The model under review builds one solid part; all positions refer to its coordinate system, in mm. A direction names the side the tool comes from. Round coordinates to 2 decimals unless told otherwise and drop trailing zeros. Order: outer loops, then holes, each group sorted by start corner. A loop starts at its lowest first (then second) coordinate and runs counter-clockwise, first axis right, second up. Notation, with made-up numbers: (-10, 71.5) - (39, 71.5) arc R10 cw to (39, 89.5) - close; hole circle Ø5 at (-29.5, -39). An arc over 180 degrees is marked (long way). One line per question, with ' | ' between items. Start each with the question number.
Item 1: For L1, parallel to Y at x = 88, z = 0.75; L2, parallel to X at y = 5, z = 1.3; L3, parallel to X at y = 3, z = 2.65, list the stretches that pass through material, from the lowest coordinate up. Write a range as [from, to].
Item 2: Tool access review of faces 1 (the face through (48, 40, 2)), 2 (the face through (37, 24, 0)), 3 (the face through (55, 20, 4)), 4 (the face through (78, 10, 2)): name each direction out of +Z, -Z, +X, -X, +Y, -Y from which nothing blocks a thin tool from reaching the whole face with its end or side.
Item 3: Add section B-B on z = 4.05. State the section outline as (x, y) points (3 decimals), and give its area (3 significant figures).
Item 4: Draft analysis for pull direction Y (two halves, no side actions). For faces 5 (the face through (13, 60, 2)), 6 (the face through (37, 24, 5)), 7 (the face through (89.3, 18.7, 2)), state which applies: +Y half, -Y half, draft (parallel to the pull), parting line (faces both ways), or undercut.
Item 5: Add section D-D on x = 54. State the section outline as (y, z) points, and give its area (3 significant figures).
Item 6: Add section C-C on y = 20. State the section outline as (x, z) points (3 decimals).
Item 7: Insertion check: pin 1 Ø1 at (x, z) = (87.5, 2.5) entering from -Y; pin 2 Ø2 at (y, z) = (20.5, 1.5) entering from -X; pin 3 Ø1.5 at (y, z) = (36, 1.5) entering from +X; pin 4 Ø1.9 at (x, y) = (88, 20) entering from -Z. Each pin has a flat end and moves straight along its axis. Give the tip position at first contact, or say it passes through.
Item 8: Add section A-A on x = 88. State the section outline as (y, z) points.
Autodesk Inventor part; units mm, degrees
ref_plane "YZ Plane" through (0, 0, 0) normal (1, 0, 0) x (0, 1, 0)
ref_plane "XZ Plane" through (0, 0, 0) normal (0, 1, 0) x (-1, 0, 0)
ref_plane "XY Plane" through (0, 0, 0) normal (0, 0, 1) x (1, 0, 0)
sketch "スケッチ1" plane through (0, 0, 0) normal (0, 0, 1) x (1, 0, 0)
  line L0 (0, 0) -> (98, 0)
  line L1 (98, 0) -> (98, 60)
  line L2 (98, 60) -> (0, 60)
  line L3 (0, 60) -> (0, 0)
  line L4 (98, 0) -> (29, 0)
  line L5 (29, 0) -> (29, 40)
  line L6 (29, 40) -> (98, 40)
  line L7 (98, 40) -> (98, 0)
  line L8 (29, 30) -> (98, 30)
  line L9 (98, 30) -> (98, 10)
  line L10 (98, 10) -> (29, 10)
  line L11 (29, 10) -> (29, 30)
  line L12 (98, 20) -> (0, 20)
  line L13 (29, 20) -> (5.906, 60)
  circle A0 centre (29, 20) radius 8.025
  circle A1 centre (14, 45.9808) radius 4.025
  line L14 (58, 40) -> (58, 0)
  line L15 (16.8756, 13) -> (-6.2184, 53)
  line L16 (41.1244, 27) -> (18.0303, 67)
  circle A2 centre (14, 45.9808) radius 14
  line L17 (16.8756, 13) -> (25.3526, -1.6825)
  point P0 (58, 30)
  point P1 (33.6188, 40)
  point P2 (22.0718, 60)
  point P3 (0, 45.9808)
  point P4 (1.8756, 38.9808)
  point P5 (24.3812, 0)
  point P6 (58, 0)
  point P7 (58, 10)
  dimension "d0" = 98
  dimension "d1" = 60
  dimension "d2" = 40
  dimension "d3" = 20
  dimension "d4" = 10
  dimension "d5" = 69
  dimension "d6" = 30
  dimension "d7" = 16.05
  dimension "d8" = 30
  dimension "d9" = 8.05
  dimension "d10" = 40
  dimension "d11" = 28
extrude "押し出し1" add sketch "スケッチ1" along normal blind 5 contours L5 L10 L14 L0 | L0 L17 L15 L12 A0 L5 | L5 A0 L12 L14 L10 | L14 L12 L1 L10 | L14 L8 L1 L12 | L12 A0 L5 L8 L14 | L15 A2 L13 A0 L12 | L8 L16 L6 L14 | A2 L13 A1 | A0 L13 A2 L16 L6 L5 | L8 L5 L6 L16 | L3 L2 L13 A2 | L13 A1 A2 | L13 L2 L16 A2
sketch "スケッチ2" plane through (0, 0, 5) normal (0, 0, 1) x (1, 0, 0)
  line L0 (98, 10) -> (98, 30)
  line L1 (98, 20) -> (47.1161, 20)
  point P0 (0, 0)
  point P1 (88, 20)
  point P2 (58, 20)
  dimension "d14" = 10
  dimension "d15" = 30
hole "穴1" at (88, 20, 5) at (58, 20, 5) direction (0, 0, -1) diameter 3.2 depth 10
fillet "フィレット1" radius 2 6 edges at (58, 40, 2.5) (58, 30, 2.5) (98, 30, 2.5) (98, 10, 2.5) (58, 0, 2.5) (58, 10, 2.5)
fillet "フィレット2" radius 10 4 edges at (24.3812, 0, 2.5) (0, 60, 2.5) (22.0718, 60, 2.5) (33.6188, 40, 2.5)
sketch "スケッチ4" plane through (0, 0, 5) normal (0, 0, 1) x (1, 0, 0)
  circle A0 centre (58, 20) radius 1.6
  circle A1 centre (58, 20) radius 3
  circle A2 centre (88, 20) radius 1.6
  circle A3 centre (88, 20) radius 3
  point P0 (0, 0)
  dimension "d34" = 6
  dimension "d35" = 6
extrude "押し出し2" cut sketch "スケッチ4" against normal blind 3 contours A0 | A1 | A2 | A3
equation "\"d35\" = d34"
properties part number "RP_Calf-Link-cover-Outside-Right"
Determined:
1) L1: [10, 18.4], [21.6, 30] | L2: [21.49, 58] | L3: [23.01, 58]
2) face 1: +Z, -Z, +X, +Y | face 2: -Z, +X, -X, +Y, -Y | face 3: +Z | face 4: +Z, -Z, +X, -Y
3) outline: (0, 45.981) arc R14 ccw to (1.876, 38.981) - (16.876, 13) - (21.494, 5) arc R10 ccw to (30.155, 0) - (56, 0) arc R2 ccw to (58, 2) - (58, 8) arc R2 cw to (60, 10) - (96, 10) arc R2 ccw to (98, 12) - (98, 28) arc R2 ccw to (96, 30) - (60, 30) arc R2 cw to (58, 32) - (58, 38) arc R2 ccw to (56, 40) - (39.392, 40) arc R10 cw to (30.732, 45) - (24.959, 55) arc R10 ccw to (16.298, 60) - (10, 60) arc R10 ccw to (0, 50) - close; hole circle Ø8.05 at (14, 45.981); hole circle Ø16.05 at (29, 20); hole circle Ø6 at (58, 20); hole circle Ø6 at (88, 20) | area: 2,820 mm2
4) face 5: +Y half | face 6: draft | face 7: undercut
5) outline: (0, 0) - (40, 0) - (40, 5) - (0, 5) - close | area: 200 mm2
6) outline: (12.834, 0) - (20.975, 0) - (20.975, 5) - (12.834, 5) - close; (37.025, 0) - (56.4, 0) - (56.4, 2) - (55, 2) - (55, 5) - (37.025, 5) - close; (59.6, 0) - (86.4, 0) - (86.4, 2) - (85, 2) - (85, 5) - (61, 5) - (61, 2) - (59.6, 2) - close; (89.6, 0) - (98, 0) - (98, 5) - (91, 5) - (91, 2) - (89.6, 2) - close
7) pin 1: y = 10 | pin 2: x = 11.97 | pin 3: x = 58 | pin 4: through
8) outline: (10, 0) - (18.4, 0) - (18.4, 2) - (17, 2) - (17, 5) - (10, 5) - close; (21.6, 0) - (30, 0) - (30, 5) - (23, 5) - (23, 2) - (21.6, 2) - close
